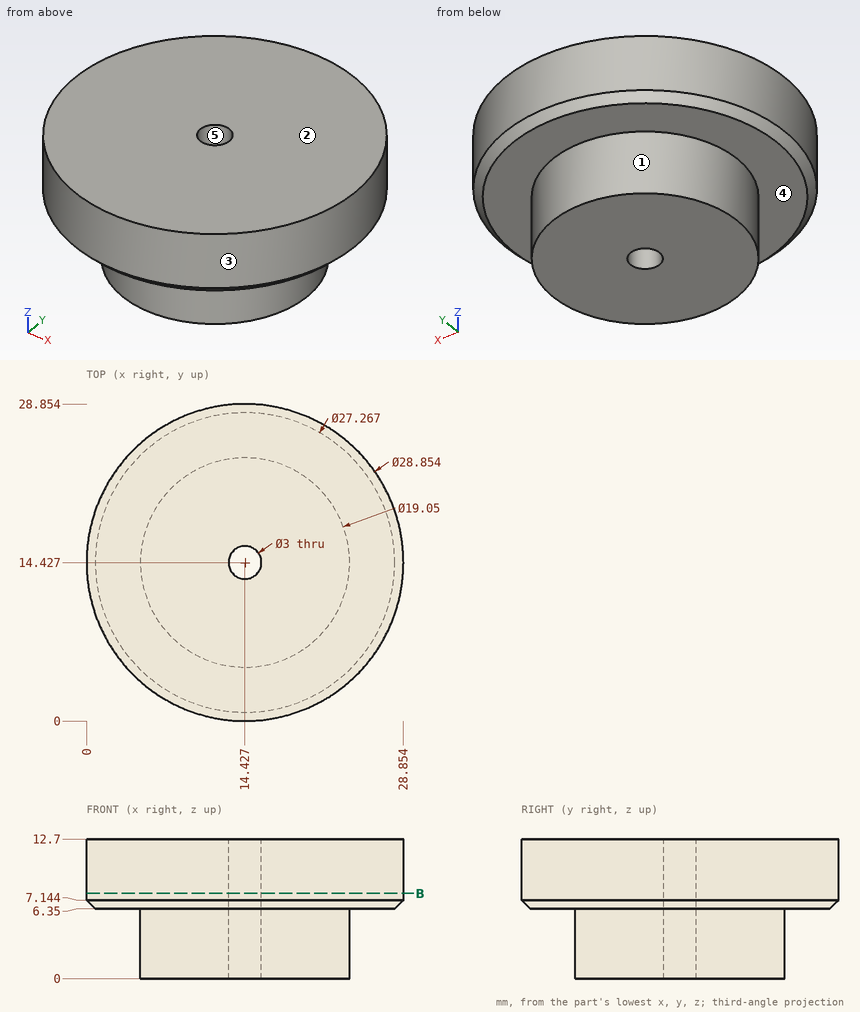
Geometry: see drawing. Coordinates: mm, zero at the bounding-box minimum. A direction names the side the tool comes from. Coordinates: 2 decimals unless noted, no trailing zeros. Write each loop counter-clockwise with the first axis right and the second up, starting at its lowest first coordinate (ties: lowest second). Pieces come first, ordered by that corner, then holes.
1) Pin query (flat end, axial travel): pin 1 Ø1.5 at (x, z) = (20.5, 7) entering from -Y; pin 2 Ø1.5 at (y, z) = (12.5, 3.5) entering from -X (1 decimal); pin 3 Ø6 at (x, z) = (18.5, 7.5) entering from +Y. Return the tip coordinate at first contact, or that it passes through.
2) Section B-B on z = 7.75. Output: boundary loops of the cut face in (x, y) (1 decimal).
3) Set-up query: the marked faces 1 and 2. Return all of +Z, -Z, +X, -X, +Y, -Y with unobstructed straight access to the full face (end or side cutting, diameter ignored); none if empty.
4) Material intervals for line 1 along Y through (x, z) = (14.5, 7) (1 decimal); line 2 along X through (y, z) = (1.5, 10) (1 decimal); line 3 along Y through (x, z) = (2, 8) (1 decimal), sorted ascending.
5) Mould query, pull axis Y, two halves, no side actions, for the marked faces 3, 4 and 5. Classes: pulls with the +Y half, pulls with the -Y half, needs draft (parallel to the pull), parting line crosses it, or undercut.
Check result:
1. pin 1: stops at y = 1.02
1. pin 2: stops at x = 5
1. pin 3: stops at y = 28.81
2. outline: circle Ø28.9 at (14.4, 14.4); hole circle Ø3 at (14.4, 14.4)
3. face 1: -Z
3. face 2: +Z, +X, -X, +Y, -Y
4. line 1: y = 0.1 to 12.9, 15.9 to 28.7
4. line 2: x = 8 to 20.8
4. line 3: y = 7.1 to 21.8
5. face 3: parting line crosses it
5. face 4: needs draft
5. face 5: undercut
